Geometry: final body of the model. Coordinates: model frame, mm. Face numbers are marked on the shaded views. Give positions to 0.01 mm unless a question says otherwise; leave off trailing zeros. Write each loop counter-clockwise with the first axis right and the second up, starting at its lowest first coordinate (ties: lowest second). Pieces come first, ordered by that corner, then holes.
Q1. Cut plane D-D on x = 5. Return the cut outline in (y, z), plus the area to 3 significant figures.
Q2. Line query: L1, parallel to X at y = 2, z = 40.5; L2, parallel to Y at x = -16, z = 67.5; L3, parallel to Y at x = 30.2, z = 55. Output: solid intervals per line, ascending.
Q3. Draft query along X for the marked faces 1, 2, 3 and 4. Return one class per face: pulls with the +X half, pulls with the -X half, needs draft (parallel to the pull), parting line crosses it, or undercut.
Q4. Cut plane A-A on y = 4.5. Return the cut outline in (x, z).
Q5. Cut plane B-B on z = 15. Return the cut outline in (x, y), plus the area to 3 significant figures.
Q6. Cut plane C-C on z = 63. Return the cut outline in (x, y), plus the area to 3 significant figures.
Q7. Pin query (flat end, axial travel): pin 1 (4 mm diameter, centred on y = 13.26, z = 55, fed in from -X); pin 2 (10 mm diameter, centred on x = -5.5, z = 23, fed in from +Y). Return the tip coordinate at first contact, or that it passes through.
```python
from build123d import *

# Parameters (mm, degrees)
SM_BASE_FLANGE_1_DEPTH   = 70
CUT_EXTRUDE_1_DEPTH      = 80.693089911
CUT_EXTRUDE_1_DEPTH_BACK = 80.693089911
SKETCH_6_R               = 2.5
CHAMFER_1_SIZE           = 5


# Sheet-metal steps are written as plain solids
with BuildPart() as part:
    # Sketch 1 → 基材-凸緣1 (new body)
    with BuildSketch(Plane.XY):
        with BuildLine():
            Line((-30, 22.5), (-30, 0.7366))
            ThreePointArc((-30, 0.7366), (-29.784254855, 0.215745145), (-29.2634, 0))
            Line((-29.2634, 0), (29.2634, 0))
            ThreePointArc((29.2634, 0), (29.784254855, 0.215745145), (30, 0.7366))
            Line((30, 0.7366), (30, 22.5))
            Line((30, 22.5), (30.7366, 22.5))
            Line((30.7366, 22.5), (30.7366, 0.7366))
            ThreePointArc((30.7366, 0.7366), (30.30510971, -0.30510971), (29.2634, -0.7366))
            Line((29.2634, -0.7366), (-29.2634, -0.7366))
            ThreePointArc((-29.2634, -0.7366), (-30.30510971, -0.30510971), (-30.7366, 0.7366))
            Line((-30.7366, 0.7366), (-30.7366, 22.5))
            Line((-30.7366, 22.5), (-30, 22.5))
        make_face()
    extrude(amount=SM_BASE_FLANGE_1_DEPTH)

    # 草圖6 → 除料-伸長1 (cut, two sides: drawn at the far end of the back side and taken through both)
    with BuildSketch(Plane(origin=(0, 0, 0), x_dir=(0, 0, -1), z_dir=(1, 0, 0)).offset(-CUT_EXTRUDE_1_DEPTH_BACK)):
        with Locations((-15, 13.2634)):
            Circle(SKETCH_6_R)
        with Locations((-55, 13.2634)):
            Circle(SKETCH_6_R)
    extrude(amount=CUT_EXTRUDE_1_DEPTH + CUT_EXTRUDE_1_DEPTH_BACK, mode=Mode.SUBTRACT)

    # 導角1
    chamfer_1_edges = [part.edges().sort_by_distance(p)[0] for p in [
        (-30.3683, 22.5, 0),
        (30.3683, 22.5, 0),
        (-30.3683, 22.5, 70),
        (30.3683, 22.5, 70),
    ]]
    chamfer(chamfer_1_edges, length=CHAMFER_1_SIZE)


solid = part.part
```
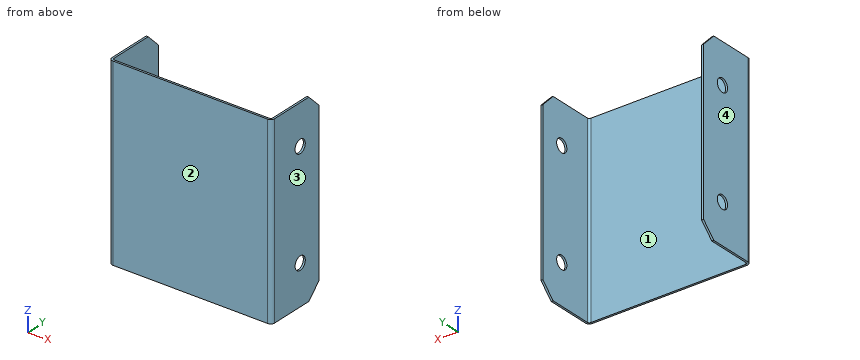
Data:
1. outline: (-0.74, 0) - (0, 0) - (0, 70) - (-0.74, 70) - close
1. area: 51.6 mm2
2. L1: x = -30.74 to -30, 30 to 30.74
2. L2: y = -0.74 to 0
2. L3: y = -0.4 to 10.76, 15.76 to 22.5
3. face 1: undercut
3. face 2: needs draft
3. face 3: pulls with the +X half
3. face 4: pulls with the -X half
4. outline: (-30.74, 0) - (-30, 0) - (-30, 70) - (-30.74, 70) - close; (30, 0) - (30.74, 0) - (30.74, 70) - (30, 70) - close
5. outline: (-30.74, 0.74) arc R1.47 ccw to (-29.26, -0.74) - (29.26, -0.74) arc R1.47 ccw to (30.74, 0.74) - (30.74, 10.76) - (30, 10.76) - (30, 0.74) arc R0.74 cw to (29.26, 0) - (-29.26, 0) arc R0.74 cw to (-30, 0.74) - (-30, 10.76) - (-30.74, 10.76) - close; (-30.74, 15.76) - (-30, 15.76) - (-30, 22.5) - (-30.74, 22.5) - close; (30, 15.76) - (30.74, 15.76) - (30.74, 22.5) - (30, 22.5) - close
5. area: 70.4 mm2
6. outline: (-30.74, 0.74) arc R1.47 ccw to (-29.26, -0.74) - (29.26, -0.74) arc R1.47 ccw to (30.74, 0.74) - (30.74, 22.5) - (30, 22.5) - (30, 0.74) arc R0.74 cw to (29.26, 0) - (-29.26, 0) arc R0.74 cw to (-30, 0.74) - (-30, 22.5) - (-30.74, 22.5) - close
6. area: 77.7 mm2
7. pin 1: passes through
7. pin 2: stops at y = 0
